The drawing under review shows one solid part. Ordinate dimensions are in mm from its lowest x, y, z. A direction names the side the tool comes from. Give positions to 0.01 mm unless a question says otherwise; leave off trailing zeros. Write each loop counter-clockwise with the first axis right and the second up, starting at its lowest first coordinate (ties: lowest second). Pieces come first, ordered by that corner, then holes. Notation, with made-up numbers: (37, 75) -> (70, 75) arc R12 ccw to (70, 92) -> close; hole circle Ø7 at (18, 52.5). An arc over 180 degrees is marked (long way). Answer as a JSON object with one key per item and string values.
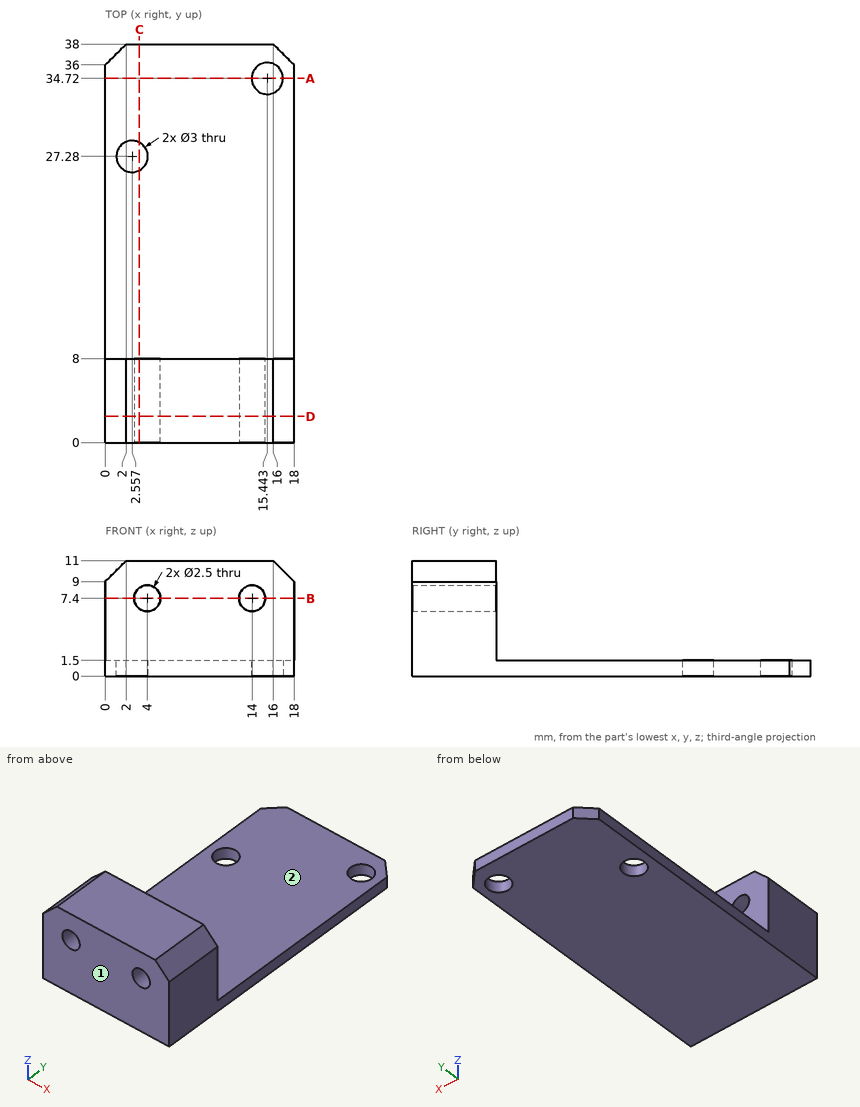
(1) We need section B-B, the plane z = 7.4. State the section outline as (x, y) points.
Here are the results:
{"outline": "(0, 0) -> (2.75, 0) -> (2.75, 8) -> (0, 8) -> close; (5.25, 0) -> (12.75, 0) -> (12.75, 8) -> (5.25, 8) -> close; (15.25, 0) -> (18, 0) -> (18, 8) -> (15.25, 8) -> close"}
(2) Clearance check with flat-ended pins moving along their axes: pin 1 (3 mm diameter, centred on x = 5.5, z = 5, fed in from +Y); pin 2 (5 mm diameter, centred on x = 15, y = 17.5, fed in from +Z); pin 3 (2 mm diameter, centred on x = 14, z = 7.4, fed in from +Y). State where each tip first meets the part, or that it passes through.
Here are the results:
{"pin 1": "stops at y = 8", "pin 2": "stops at z = 1.5", "pin 3": "passes through"}
(3) We need section C-C, the plane x = 3.25. State the section outline as (y, z) points.
Here are the results:
{"outline": "(0, 0) -> (25.95, 0) -> (25.95, 1.5) -> (8, 1.5) -> (8, 6.4) -> (0, 6.4) -> close; (0, 8.4) -> (8, 8.4) -> (8, 11) -> (0, 11) -> close; (28.61, 0) -> (38, 0) -> (38, 1.5) -> (28.61, 1.5) -> close"}
(4) We need section D-D, the plane y = 2.5. State the section outline as (x, z) points.
Here are the results:
{"outline": "(0, 0) -> (18, 0) -> (18, 9) -> (16, 11) -> (2, 11) -> (0, 9) -> close; hole circle Ø2.5 at (4, 7.4); hole circle Ø2.5 at (14, 7.4)"}
(5) We need section A-A, the plane y = 34.72. State the section outline as (x, z) points.
Here are the results:
{"outline": "(0, 0) -> (13.94, 0) -> (13.94, 1.5) -> (0, 1.5) -> close; (16.94, 0) -> (18, 0) -> (18, 1.5) -> (16.94, 1.5) -> close"}
(6) For the marked faces 1 and 2, list the 3-axis set-ups (+Z, -Z, +X, -X, +Y, -Y) from which the entire face can be reached by the end or side of a thin tool; tool diameter is ignored.
Here are the results:
{"face 1": "+Z, -Z, +X, -X, -Y", "face 2": "+Z, +X, -X, +Y"}
(7) For line 1 along X through (y, z) = (5.75, 7.4); line 2 along Z through (x, y) = (4, 6.25); line 3 along Y through (x, z) = (12, 5.5), list the stretches that pass through material, from the lowest coordinate up.
Here are the results:
{"line 1": "x = 0 to 2.75, 5.25 to 12.75, 15.25 to 18", "line 2": "z = 0 to 6.15, 8.65 to 11", "line 3": "y = 0 to 8"}
